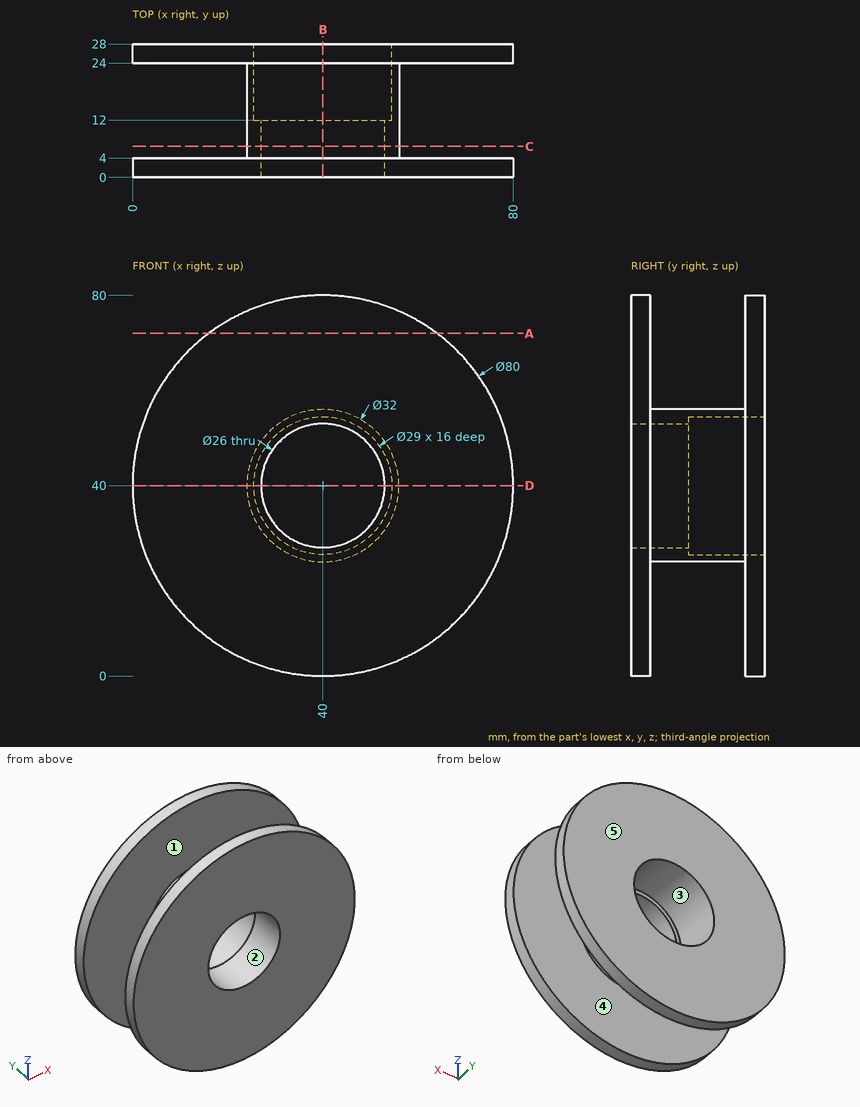
Source: three-view drawing plus pictorial views. Frame: mm from the lowest corner of the part. A direction names the side the tool comes from. Round coordinates to 2 decimals unless told otherwise and drop trailing zeros. Loops run counter-clockwise (first coordinate to the right, second up) from the corner with the lowest first, then second, coordinate; pieces in that order, holes last.
1. Section query C-C on y = 6.5. Output: boundary loops of the cut face in (x, z), and give its area (3 significant figures).
2. Mould query, pull axis X, two halves, no side actions, for the marked faces 1 and 2. Classes: released by +X, released by -X, zero draft, split by the parting line, or undercut.
3. Contact query for flat-ended pins moving along their axis: pin 1 (1 mm diameter, centred on x = 32, z = 50.5, fed in from +Y); pin 2 (5 mm diameter, centred on y = 12.5, z = 39.5, fed in from -X); pin 3 (10 mm diameter, centred on x = 47.5, y = 18.5, fed in from +Z); pin 4 (23.5 mm diameter, centred on x = 40, z = 40, fed in from +Y). Output: stop coordinate, or through.
4. Section query B-B on x = 40. Output: boundary loops of the cut face in (y, z), and give its area (3 significant figures).
5. Section query A-A on z = 72. Output: boundary loops of the cut face in (x, y).
6. Section query D-D on z = 40. Output: boundary loops of the cut face in (x, y), and give its area (3 significant figures).
7. Access query for the marked faces 3, 4 and 5. Directions: +Z, -Z, +X, -X, +Y, -Y. A direction counts if a zero-diameter tool reaches every point of the face in a straight line with its end or side. Return the directions, or none.
8. Ray query, L1, parallel to Y at x = 32, z = 72; L2, parallel to Z at x = 40, y = 6.5; L3, parallel to X at y = 15.5, z = 40. Return the intervals inside material, ascending.
Answers below:
1. outline: circle Ø32 at (40, 40); hole circle Ø26 at (40, 40)
1. area: 273 mm2
2. face 1: zero draft
2. face 2: undercut
3. pin 1: stops at y = 12
3. pin 2: stops at x = 24
3. pin 3: stops at z = 55.8
3. pin 4: passes through
4. outline: (0, 0) - (4, 0) - (4, 24) - (24, 24) - (24, 0) - (28, 0) - (28, 25.5) - (12, 25.5) - (12, 27) - (0, 27) - close; (0, 53) - (12, 53) - (12, 54.5) - (28, 54.5) - (28, 80) - (24, 80) - (24, 56) - (4, 56) - (4, 80) - (0, 80) - close
4. area: 504 mm2
5. outline: (16, 0) - (64, 0) - (64, 4) - (16, 4) - close; (16, 24) - (64, 24) - (64, 28) - (16, 28) - close
6. outline: (0, 0) - (27, 0) - (27, 12) - (25.5, 12) - (25.5, 28) - (0, 28) - (0, 24) - (24, 24) - (24, 4) - (0, 4) - close; (53, 0) - (80, 0) - (80, 4) - (56, 4) - (56, 24) - (80, 24) - (80, 28) - (54.5, 28) - (54.5, 12) - (53, 12) - close
6. area: 504 mm2
7. face 3: +Y
7. face 4: none
7. face 5: +Z, -Z, +X, -X, +Y
8. L1: y = 0 to 4, 24 to 28
8. L2: z = 24 to 27, 53 to 56
8. L3: x = 24 to 25.5, 54.5 to 56
